from build123d import *

# Parameters (mm, degrees)
MODEL_W             = 5.5
MODEL_H             = 5.5
BOSS_EXTRUDE1_DEPTH = 6


with BuildPart() as part:
    # Model → Boss-Extrude1 (new body)
    with BuildSketch(Plane.XY):
        with BuildLine():
            Line((2982.612369189, 1260.808846123), (2982.612369189, 1221.808846123))
            Line((2982.612369189, 1221.808846123), (2995.112369189, 1221.808846123))
            Line((2995.112369189, 1221.808846123), (2995.112369189, 1215.808846123))
            Line((2995.112369189, 1215.808846123), (3001.112369189, 1215.808846123))
            Line((3001.112369189, 1215.808846123), (3001.112369189, 1221.808846123))
            Line((3001.112369189, 1221.808846123), (3003.612369189, 1221.808846123))
            Line((3003.612369189, 1221.808846123), (3003.612369189, 1252.808846123))
            Line((3003.612369189, 1252.808846123), (2992.612369189, 1252.808846123))
            Line((2992.612369189, 1252.808846123), (2992.612369189, 1260.808846123))
            ThreePointArc((2992.612369189, 1260.808846123), (3033.612369189, 1301.808846123), (3074.612369189, 1260.808846123))
            Line((3074.612369189, 1260.808846123), (3074.612369189, 1252.808846123))
            Line((3074.612369189, 1252.808846123), (3063.612369189, 1252.808846123))
            Line((3063.612369189, 1252.808846123), (3063.612369189, 1221.808846123))
            Line((3063.612369189, 1221.808846123), (3074.612369189, 1221.808846123))
            Line((3074.612369189, 1221.808846123), (3084.612369189, 1221.808846123))
            Line((3084.612369189, 1221.808846123), (3084.612369189, 1260.808846123))
            ThreePointArc((3084.612369189, 1260.808846123), (3033.612369189, 1311.808846123), (2982.612369189, 1260.808846123))
        make_face()
        with Locations((3069.112369189, 1227.308846123)):
            Rectangle(MODEL_W, MODEL_H, mode=Mode.SUBTRACT)
        with Locations((3069.112369189, 1247.308846123)):
            Rectangle(MODEL_W, MODEL_H, mode=Mode.SUBTRACT)
        with Locations((2998.112369189, 1227.308846123)):
            Rectangle(MODEL_W, MODEL_H, mode=Mode.SUBTRACT)
        with Locations((2998.112369189, 1247.308846123)):
            Rectangle(MODEL_W, MODEL_H, mode=Mode.SUBTRACT)
    extrude(amount=BOSS_EXTRUDE1_DEPTH)


solid = part.part
The listing builds one solid part. Answer for the finished solid, in the listing's coordinates (mm). A direction names the side the tool comes from. Round coordinates to 2 decimals unless told otherwise and drop trailing zeros. Order: outer loops, then holes, each group sorted by start corner. A loop starts at its lowest first (then second) coordinate and runs counter-clockwise, first axis right, second up. Notation, with made-up numbers: (57.5, -10.75) -> (111.5, -10.75) arc R12 ccw to (111.5, 1.25) -> close; hole circle Ø7 at (-21, 85.5). An arc over 180 degrees is marked (long way). One line per item, written item: value.
Item 1: Find section A-A, the plane y = 1227. Give the vertices of the cut face in (x, z), then the cut area to 3 significant figures.
Taken from the geometry:
outline: (2982.61, 0) -> (2995.36, 0) -> (2995.36, 6) -> (2982.61, 6) -> close; (3000.86, 0) -> (3003.61, 0) -> (3003.61, 6) -> (3000.86, 6) -> close; (3063.61, 0) -> (3066.36, 0) -> (3066.36, 6) -> (3063.61, 6) -> close; (3071.86, 0) -> (3084.61, 0) -> (3084.61, 6) -> (3071.86, 6) -> close
area: 186 mm2
Item 2: Straight lines are drawn through the part: L1, parallel to X at y = 1236.5, z = 4.85; L2, parallel to Y at x = 3071, z = 1.8; L3, parallel to X at y = 1259.5, z = 0.7. For each, find the intervals that lie inside material, in ascending order.
Taken from the geometry:
L1: x = 2982.61 to 3003.61, 3063.61 to 3084.61
L2: y = 1221.81 to 1224.56, 1230.06 to 1244.56, 1250.06 to 1252.81, 1277.64 to 1295.5
L3: x = 2982.61 to 2992.61, 3074.61 to 3084.61
Item 3: For a pull along X with two mould halves and no side action, classify faces 6 (the cylindrical face through (3032.7, 1301.8, 3)), 7 (the flat face through (3006.9, 1292.5, 0)), 8 (the flat face through (2982.612, 1242, 3)) as released by +X, released by -X, zero draft, split by the parting line, or undercut.
Taken from the geometry:
face 6: undercut
face 7: zero draft
face 8: released by -X
Item 4: Find section C-C, the plane z = 3.7. State how many separate pieces and enclosed holes the cut face has, then the cut area to 3 significant figures.
Taken from the geometry:
separate pieces: 1
enclosed holes: 4
area: 2,820 mm2
Item 5: For faces 1 (the flat face through (3003.612, 1237, 3)), 2 (the flat face through (2995.362, 1247, 3)), 3 (the flat face through (2998, 1215.809, 3)), 4 (the flat face through (2989, 1221.809, 3)), 5 (the flat face through (3001.112, 1219, 3)), determine the directions among +Z, -Z, +X, -X, +Y, -Y from which every point of the face is accessible in a straight line to the end or side of a thin tool.
Taken from the geometry:
face 1: +Z, -Z, -Y
face 2: +Z, -Z
face 3: +Z, -Z, +X, -X, -Y
face 4: +Z, -Z, -X, -Y
face 5: +Z, -Z, +X, -Y
Item 6: Given P1, Ø1.8, axis at y = 1219, z = 2.5, coming from the -X side; P2, Ø1.6, axis at x = 3069, z = 3, coming from the +Y side; P3, Ø3, axis at x = 3070, z = 3.5, coming from the +Y side, each flat-ended and moving along its own axis, determine where each tip first touches the part or whether it passes through.
Taken from the geometry:
P1: stops at x = 2995.11
P2: stops at y = 1298.29
P3: stops at y = 1298.01
Item 7: Find section B-B, the plane y = 1285.5. Give the vertices of the cut face in (x, z).
Taken from the geometry:
outline: (2988.99, 0) -> (3000.88, 0) -> (3000.88, 6) -> (2988.99, 6) -> close; (3066.34, 0) -> (3078.24, 0) -> (3078.24, 6) -> (3066.34, 6) -> close
Item 8: Find section D-D, the plane y = 1242.5. Give the vertices of the cut face in (x, z).
Taken from the geometry:
outline: (2982.61, 0) -> (3003.61, 0) -> (3003.61, 6) -> (2982.61, 6) -> close; (3063.61, 0) -> (3084.61, 0) -> (3084.61, 6) -> (3063.61, 6) -> close
